Verification items for the finished model (mm, model axes). Face numbers are marked on the shaded views. A direction names the side the tool comes from. Round coordinates to 2 decimals unless told otherwise and drop trailing zeros. Order: outer loops, then holes, each group sorted by start corner. A loop starts at its lowest first (then second) coordinate and runs counter-clockwise, first axis right, second up. Notation, with made-up numbers: M 35,0.5 L 79,0.5 A23 ccw 79,17.5 Z; hole C -13.5,61 d10. An arc over 180 degrees is marked long. Use CSV: the item, a comma, the result in double quotes. Start each with the question number.
Q1. Sectioned sample at C-C (z = 16.25). Enter the section's corners in (x, y), and give its area (3 significant figures).
Q2. Scan lines: line 1 (X direction, y = -12.5, z = 19.25); line 2 (Y direction, x = -2, z = 14); line 3 (X direction, y = 10, z = 4.5). Record each from-to range of solid material in increasing order.
Q3. Gauge pin test, flat ends, axial feed: pin 1 Ø5 at (y, z) = (-3.5, 15) entering from -X; pin 2 Ø6 at (x, z) = (14, 8.5) entering from -Y; pin 3 Ø4.5 at (x, z) = (13, 10) entering from +Y. Record the tip position at first contact, or that the pin passes through.
Q4. Set-up check for the marked faces 5 and 6: record each of +Z, -Z, +X, -X, +Y, -Y from which the full face is reachable in a straight line by a thin tool's end or side.
Q5. Mould release check, pull along Y, two halves, no side actions. Record for the marked faces 1, 2, 3 and 4: +Y half, -Y half, draft (parallel to the pull), parting line (faces both ways), or undercut.
```python
from build123d import *

# Parameters (mm, degrees)
F0_W     = 90
F0_H     = 70
F0_W_2   = 82
F0_H_2   = 60
F1_DEPTH = 5
F2_DEPTH = 20
F3_DEPTH = 20
F4_R     = 4.99999


# Not quite as in the source:
# - a fillet or chamfer is up to 0.001 mm smaller than in the source, because OpenCascade refuses the exact size
# - a feature names something its author has since deleted; it is built from what else it names


with BuildPart() as f1:
    # F0 (on Top) → F1 (new body)
    with BuildSketch(Plane.XY):
        with BuildLine():
            Line((-50, -50), (50, -50))
            ThreePointArc((50, -50), (57.0710678119, -47.0710678119), (60, -40))
            Line((60, -40), (60, 40))
            ThreePointArc((60, 40), (57.0710678119, 47.0710678119), (50, 50))
            Line((50, 50), (-50, 50))
            ThreePointArc((-50, 50), (-57.0710678119, 47.0710678119), (-60, 40))
            Line((-60, 40), (-60, -40))
            ThreePointArc((-60, -40), (-57.0710678119, -47.0710678119), (-50, -50))
        make_face()
        Rectangle(F0_W, F0_H, mode=Mode.SUBTRACT)
        Rectangle(F0_W, F0_H)
        Rectangle(F0_W_2, F0_H_2, mode=Mode.SUBTRACT)
    extrude(amount=F1_DEPTH)

    # F0 (on Top) → F2 (join)
    with BuildSketch(Plane.XY):
        Rectangle(F0_W, F0_H)
        Rectangle(F0_W_2, F0_H_2, mode=Mode.SUBTRACT)
        Rectangle(F0_W_2, F0_H_2)
    extrude(amount=F2_DEPTH)

    # F0 (on Top) → F3 (cut)
    with BuildSketch(Plane.XY):
        Rectangle(F0_W_2, F0_H_2)
    extrude(amount=F3_DEPTH, mode=Mode.SUBTRACT)

    # F4 (radius 5 in the source; OpenCascade refuses exactly that, so slightly less here)
    f4_edges = [f1.edges().sort_by_distance(p)[0] for p in [
        (57.071068, -47.071068, 0),
    ]]
    fillet(f4_edges, radius=F4_R)


solid = f1.part
```
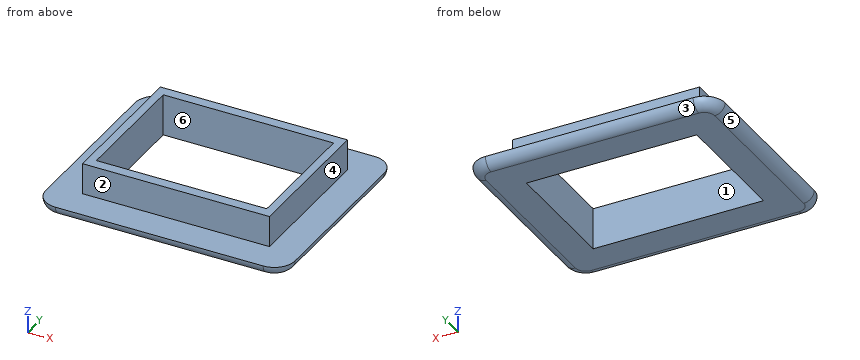
Verdict:
1,outline,"M -45,-35 L 45,-35 L 45,35 L -45,35 Z; hole M -41,-30 L 41,-30 L 41,30 L -41,30 Z"
1,area,"1,380 mm²"
2,line 1,"x = -45 to -41, 41 to 45"
2,line 2,"y = -35 to -30, 30 to 35"
2,line 3,"x = -59.97 to -41, 41 to 59.97"
3,pin 1,"stops at x = -45"
3,pin 2,"stops at y = -35"
3,pin 3,"stops at y = 35"
4,face 5,"-Z, -X, +Y, -Y"
4,face 6,"+Z, -Z"
5,face 1,"undercut"
5,face 2,"-Y half"
5,face 3,"+Y half"
5,face 4,"draft"
